The listing builds one solid part. Answer for the finished solid, in the listing's coordinates (mm). Give positions to 0.01 mm unless a question says otherwise; leave off trailing zeros. Loops run counter-clockwise (first coordinate to the right, second up) from the corner with the lowest first, then second, coordinate; pieces in that order, holes last. Notation, with made-up numbers: (83, 70) - (107, 70) arc R16 cw to (107, 95) - close; hole circle Ø1 at (38, 20). An arc over 180 degrees is marked (long way). Write item = value, one per line. Start each with the question number.
1) The part is cut by section A-A on y = 100. Write down the section's boundary in (x, z).
2) The part is cut by section B-B on x = -21.5. Write down the section's boundary in (y, z), plus the area to 3 significant figures.
3) The mould has two halves that part along Y. Classify faces 1 (the cylindrical face through (95.52, 33.965, 1.521)), 2 (the flat face through (-2, 76, 3)): +Y half, -Y half, draft (parallel to the pull), parting line (faces both ways), or undercut.
4) The part is cut by section C-C on x = 117.6. Write down the section's boundary in (y, z), plus the area to 3 significant figures.
5) The part is cut by section D-D on z = 0.9. State how many separate pieces and enclosed holes the cut face has, plus the area to 3 significant figures.
6) Consider probe 1 along X at (y, z) = (27.5, 2.1); probe 2 along Y at (x, z) = (-10.88, 1); probe 3 along X at (y, z) = (109.12, 1.9). Determine where each line is inside the solid, lowest interval first.
from build123d import *

# Parameters (mm, degrees)
SKETCH_2_W          = 350
SKETCH_2_H          = 150
EXTRUDE_1_DEPTH     = 3
SKETCH_3_R          = 3
SKETCH_3_R_2        = 3.5
SKETCH_3_R_3        = 1.25
SKETCH_3_R_4        = 7.75
SKETCH_3_W          = 31.7
SKETCH_3_H          = 25.4
SKETCH_3_W_2        = 13
SKETCH_3_H_2        = 19
CUT_EXTRUDE_1_DEPTH = 231.508134347


with BuildPart() as part:
    # 草图2 → 凸台-拉伸1 (new body)
    with BuildSketch(Plane.XY):
        with Locations((0, 75)):
            Rectangle(SKETCH_2_W, SKETCH_2_H)
    extrude(amount=EXTRUDE_1_DEPTH)

    # 草图3 → 切除-拉伸1 (cut, through all)
    with BuildSketch(Plane.XY.offset(3)):
        with Locations((40.5, 30.875)):
            Circle(SKETCH_3_R)
        with Locations((65.5, 30.875)):
            Circle(SKETCH_3_R)
        with Locations((80.6, 31.6)):
            Circle(SKETCH_3_R_2)
        with Locations((98.1, 31.6)):
            Circle(SKETCH_3_R_2)
        with Locations((117.6, 31.6)):
            Circle(SKETCH_3_R_2)
        with Locations((131.6, 31.6)):
            Circle(SKETCH_3_R_2)
        with Locations((-149.12, 109.12)):
            Circle(SKETCH_3_R_3)
        with Locations((-130.88, 109.12)):
            Circle(SKETCH_3_R_3)
        with Locations((-149.12, 90.88)):
            Circle(SKETCH_3_R_3)
        with Locations((-130.88, 90.88)):
            Circle(SKETCH_3_R_3)
        with Locations((-140, 100)):
            Circle(SKETCH_3_R_4)
        with Locations((-29.12, 90.88)):
            Circle(SKETCH_3_R_3)
        with Locations((-10.88, 90.88)):
            Circle(SKETCH_3_R_3)
        with Locations((-20, 100)):
            Circle(SKETCH_3_R_4)
        with Locations((-29.12, 109.12)):
            Circle(SKETCH_3_R_3)
        with Locations((-10.88, 109.12)):
            Circle(SKETCH_3_R_3)
        with Locations((65.5, 49.925)):
            Circle(SKETCH_3_R)
        with Locations((40.5, 49.925)):
            Circle(SKETCH_3_R)
        with BuildLine():
            Line((61.75, 45.925), (61.75, 53.925))
            ThreePointArc((61.75, 53.925), (61.457106781, 54.632106781), (60.75, 54.925))
            Line((60.75, 54.925), (45.25, 54.925))
            ThreePointArc((45.25, 54.925), (44.542893219, 54.632106781), (44.25, 53.925))
            Line((44.25, 53.925), (44.25, 45.925))
            ThreePointArc((44.25, 45.925), (44.542893219, 45.217893219), (45.25, 44.925))
            Line((45.25, 44.925), (60.75, 44.925))
            ThreePointArc((60.75, 44.925), (61.457106781, 45.217893219), (61.75, 45.925))
        make_face()
        with BuildLine():
            Line((45.25, 25.875), (60.75, 25.875))
            ThreePointArc((60.75, 25.875), (61.457106781, 26.167893219), (61.75, 26.875))
            Line((61.75, 26.875), (61.75, 34.875))
            ThreePointArc((61.75, 34.875), (61.457106781, 35.582106781), (60.75, 35.875))
            Line((60.75, 35.875), (45.25, 35.875))
            ThreePointArc((45.25, 35.875), (44.542893219, 35.582106781), (44.25, 34.875))
            Line((44.25, 34.875), (44.25, 26.875))
            ThreePointArc((44.25, 26.875), (44.542893219, 26.167893219), (45.25, 25.875))
        make_face()
        with Locations((-139.15, 28.7)):
            Rectangle(SKETCH_3_W, SKETCH_3_H)
        with Locations((-106.8, 28.7)):
            Rectangle(SKETCH_3_W_2, SKETCH_3_H_2)
    extrude(amount=-CUT_EXTRUDE_1_DEPTH, mode=Mode.SUBTRACT)


solid = part.part
Answer below:
q1.outline = (-175, 0) - (-147.75, 0) - (-147.75, 3) - (-175, 3) - close; (-132.25, 0) - (-27.75, 0) - (-27.75, 3) - (-132.25, 3) - close; (-12.25, 0) - (175, 0) - (175, 3) - (-12.25, 3) - close
q2.outline = (0, 0) - (92.4, 0) - (92.4, 3) - (0, 3) - close; (107.6, 0) - (150, 0) - (150, 3) - (107.6, 3) - close
q2.area = 404 mm2
q3.face_1 = undercut
q3.face_2 = draft
q4.outline = (0, 0) - (28.1, 0) - (28.1, 3) - (0, 3) - close; (35.1, 0) - (150, 0) - (150, 3) - (35.1, 3) - close
q4.area = 429 mm2
q5.separate_pieces = 1
q5.enclosed_holes = 22
q5.area = 50,400 mm2
q6.probe_1 = -175 to -155, -123.3 to -113.3, -100.3 to 44.25, 61.75 to 175
q6.probe_2 = 0 to 89.63, 92.13 to 107.87, 110.37 to 150
q6.probe_3 = -175 to -150.37, -147.87 to -132.13, -129.63 to -30.37, -27.87 to -12.13, -9.63 to 175
